Check sheet for the modelled part. Datum: model origin and axes. Units: mm. A direction names the side the tool comes from. Give positions to 0.01 mm unless a question says otherwise; leave off trailing zeros. Loops run counter-clockwise (first coordinate to the right, second up) from the corner with the lowest first, then second, coordinate; pieces in that order, holes last. Notation, with made-up numbers: M 48.5,47.25 L 89.5,47.25 A16 ccw 89.5,67.25 Z; hole C 65,-6 d6. An arc over 180 degrees is marked long. One line per question, with ' | ' between items. Start each with the question number.
Autodesk Inventor part; units mm, degrees
ref_plane "YZ Plane" through (0, 0, 0) normal (1, 0, 0) x (0, 1, 0)
ref_plane "XZ Plane" through (0, 0, 0) normal (0, 1, 0) x (-1, 0, 0)
ref_plane "XY Plane" through (0, 0, 0) normal (0, 0, 1) x (1, 0, 0)
sketch "Sketch1" plane through (0, 0, 0) normal (0, 0, 1) x (1, 0, 0)
  circle A0 centre (0, 0) radius 11.5
  line L0 (-26, 4.25) -> (26, 4.25)
  line L1 (26, 4.25) -> (26, -4.25)
  line L2 (26, -4.25) -> (-26, -4.25)
  line L3 (-26, -4.25) -> (-26, 4.25)
  point P0 (-26, 0)
  point P1 (0, 4.25)
  dimension "d0" = 23
  dimension "d1" = 52
  dimension "d2" = 8.5
extrude "Extrusion1" add sketch "Sketch1" along normal blind 2 contours A0 L2 L0 | A0 L0 L1 L2 | A0 L2 L3 L0
extrude "Extrusion2" add sketch "Sketch1" along normal blind 17.9 contours A0 L2 L0 | L0 A0 | A0 L2
sketch "Sketch2" plane through (0, 0, 0) normal (0, 0, 1) x (1, 0, 0)
  line L0 (-27.9259, 0) -> (33.5172, 0) construction
  point P0 (0, 0)
  point P1 (-23, 0)
  point P2 (23, 0)
  dimension "d7" = 0
  dimension "d8" = 23
  dimension "d9" = 23
hole "Hole1" at (-23, 0, 0) at (23, 0, 0) direction (0, 0, 1) diameter 2.7178 end through all
fillet "Fillet1" radius 1.905 4 edges at (-26, -4.25, 1) (26, -4.25, 1) (26, 4.25, 1) (-26, 4.25, 1)
fillet "Fillet2" radius 0.635 1 edges at (-11.5, 0, 17.9)
hole "Hole2" at (0, 0, 0) direction (0, 0, 1) diameter 8.89 depth 12.7 tip angle 118
properties material "FR4"
Q1. Access from +Z, -Z, +X, -X, +Y, -Y to the whole of each face (thin tool, end or side, straight path). Record for faces 5 (the flat face through (17, 4.25, 1)), 6 (the cylindrical face through (-2.493, 11.227, 8.512)), 7 (the flat face through (17, -4.25, 1)), 8 (the cylindrical face through (4.34, -0.96, 6.44)), 9 (the flat face through (-17, -4.25, 1)).
Q2. Material ranges on probe 1 along Y at (x, z) = (23, 1.4); probe 2 along Z at (x, y) = (-22.5, 2.75); probe 3 along X at (y, z) = (-0.25, 16.75), recorded low to high. Write a range as from..to.
Q3. Cross-section at C-C (x = -12). Record the cut outline in (y, z).
Q4. Depth check by flat-ended pin: P1, Ø1, axis at x = 18, z = 1.5, coming from the -Y side; P2, Ø8, axis at y = 7, z = 9, coming from the -X side; P3, Ø1, axis at y = -1, z = 7.5, coming from the +X side; P4, Ø2.5, axis at x = -23, y = 0, coming from the +Z side. Enter the tip coordinate at first touch or a pass-through.
Q5. Cross-section at B-B (z = 8.5). Record the cut outline in (x, y) (3 decimals), and give its area (3 significant figures).
Q6. Cross-section at D-D (z = 13.5). Record the cut outline in (x, y).
Q7. Draft check along X on faces 1 (the flat face through (18, 0, 2)), 2 (the cylindrical face through (-25.427, 3.707, 1.014)), 3 (the conical face through (-0.75, -0.17, 14.91)), 4 (the cylindrical face through (-24.347, -0.177, 1.014)). Enter one of: released by +X, released by -X, zero draft, split by the parting line, or undercut.
Q8. Cross-section at A-A (x = 23). Record the cut outline in (y, z).
Solved:
1) face 5: +Z, -Z, +X, +Y | face 6: +Z | face 7: +Z, -Z, +X, -Y | face 8: -Z | face 9: +Z, -Z, -X, -Y
2) probe 1: y = -4.25..-1.36, 1.36..4.25 | probe 2: z = 0..2 | probe 3: x = -11.5..11.5
3) outline: M -4.25,0 L 4.25,0 L 4.25,2 L -4.25,2 Z
4) P1: stops at y = -4.25 | P2: stops at x = -11.1 | P3: stops at x = 11.49 | P4: passes through
5) outline: C 0,0 d23; hole C 0,0 d8.89 | area: 353 mm²
6) outline: C 0,0 d23; hole C 0,0 d6.23
7) face 1: zero draft | face 2: released by -X | face 3: undercut | face 4: undercut
8) outline: M -4.25,0 L -1.36,0 L -1.36,2 L -4.25,2 Z; M 1.36,0 L 4.25,0 L 4.25,2 L 1.36,2 Z
